Build history of the part. All positions in model axes, mm. Face numbers are marked on the shaded views. Coordinates: 2 decimals unless noted, no trailing zeros. Return JSON: item names as keys, results as strings.
from build123d import *

# Parameters (mm, degrees)
F0_R     = 2
F1_DEPTH = 15
F2_R     = 2
F3_SIZE2 = 0.334
F3_SIZE  = 0.167
F4_R     = 0.5
F5_SIZE  = 0.334


with BuildPart() as f1:
    # F0 (on Top) → F1 (new body)
    with BuildSketch(Plane.XY):
        with BuildLine():
            ThreePointArc((0, 7.5), (6.509248113, 3.7255454638), (6.4667999415, -3.7987495992))
            Line((6.4667999415, -3.7987495992), (7.3290399337, -4.3052495457))
            ThreePointArc((7.3290399337, -4.3052495457), (8.4999852198, -0.0158512782), (7.3450462726, 4.2778844366))
            ThreePointArc((7.3450462726, 4.2778844366), (10.1862523655, 11.2386714824), (3.53743112, 7.7289443698))
            ThreePointArc((3.53743112, 7.7289443698), (1.8102448532, 8.304999312), (0, 8.5))
            Line((0, 8.5), (0, 7.5))
        make_face()
        with Locations((7.5, 8.2748819776)):
            Circle(F0_R, mode=Mode.SUBTRACT)
        with BuildLine():
            ThreePointArc((-6.4667999415, -3.7987495992), (-6.509248113, 3.7255454638), (0, 7.5))
            Line((0, 7.5), (0, 8.5))
            ThreePointArc((0, 8.5), (-1.8102448532, 8.304999312), (-3.53743112, 7.7289443698))
            ThreePointArc((-3.53743112, 7.7289443698), (-10.1862523655, 11.2386714824), (-7.3450462726, 4.2778844366))
            ThreePointArc((-7.3450462726, 4.2778844366), (-8.4999852198, -0.0158512782), (-7.3290399337, -4.3052495457))
            Line((-7.3290399337, -4.3052495457), (-6.4667999415, -3.7987495992))
        make_face()
        with Locations((-7.5, 8.2748819776)):
            Circle(F0_R, mode=Mode.SUBTRACT)
    extrude(amount=F1_DEPTH)

    # F2
    f2_edges = [f1.edges().sort_by_distance(p)[0] for p in [
        (7.345046, 4.277884, 7.5),
        (3.537431, 7.728944, 7.5),
        (-3.537431, 7.728944, 7.5),
        (-7.345046, 4.277884, 7.5),
    ]]
    fillet(f2_edges, radius=F2_R)

    # F3
    f3_edges = [f1.edges().sort_by_distance(p)[0] for p in [
        (8.431287, -1.078612, 0),
        (8.276969, 3.688682, 0),
        (6.89792, -4.052, 0),
        (10.186252, 11.238671, 0),
        (0, 7.5, 0),
        (2.859731, 8.598635, 0),
        (-6.89792, -4.052, 0),
        (0, 8.5, 0),
        (-8.431287, -1.078612, 0),
        (-2.859731, 8.598635, 0),
        (-8.276969, 3.688682, 0),
        (-10.186252, 11.238671, 0),
        (5.5, 8.274882, 0),
        (-9.5, 8.274882, 0),
    ]]
    f3_side = f1.faces().sort_by_distance((8.150047, -1.042633, 0))[0]
    chamfer(f3_edges, length=F3_SIZE, length2=F3_SIZE2, reference=f3_side)

    # F4
    f4_edges = [f1.edges().sort_by_distance(p)[0] for p in [
        (-7.32904, -4.30525, 7.667),
        (7.32904, -4.30525, 7.667),
    ]]
    fillet(f4_edges, radius=F4_R)

    # F5
    f5_edges = [f1.edges().sort_by_distance(p)[0] for p in [
        (8.460888, -0.814478, 15),
        (7.278526, -4.092712, 15),
        (8.276969, 3.688682, 15),
        (6.675617, -3.921414, 15),
        (10.186252, 11.238671, 15),
        (0, 7.5, 15),
        (2.859731, 8.598635, 15),
        (-6.675617, -3.921414, 15),
        (0, 8.5, 15),
        (-7.278526, -4.092712, 15),
        (-2.859731, 8.598635, 15),
        (-8.460888, -0.814478, 15),
        (-10.186252, 11.238671, 15),
        (-8.276969, 3.688682, 15),
        (5.5, 8.274882, 15),
        (-9.5, 8.274882, 15),
    ]]
    chamfer(f5_edges, length=F5_SIZE)


solid = f1.part
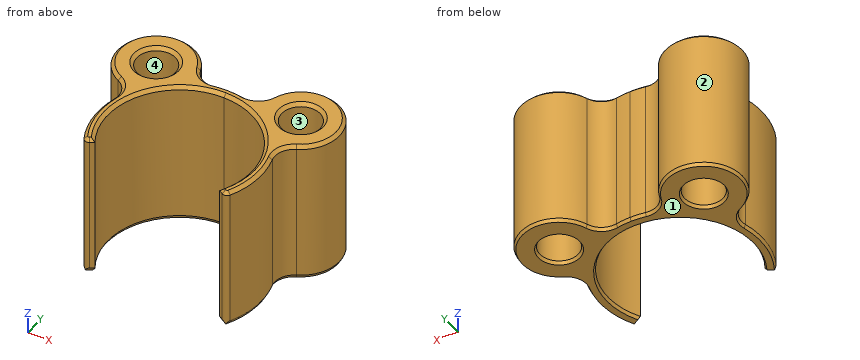
1. Probe L1, parallel to X at y = 11.75, z = 13.5; L2, parallel to X at y = 11.5, z = 7.5; L3, parallel to Y at x = 2.5, z = 12. List the from-to ranges inside material, lowest first.
Check values:
{"L1": "-9.48 to -5.52, 5.52 to 9.48", "L2": "-9.87 to -5.13, 5.13 to 9.87", "L3": "7.07 to 8.44"}
2. Drop flat-ended pins along their axis: pin 1 (1 mm diameter, centred on x = 1, z = 7, fed in from +Y); pin 2 (6 mm diameter, centred on x = -5.5, y = 9, fed in from +Z); pin 3 (3.5 mm diameter, centred on x = -7.5, y = 8.27, fed in from +Z). Give the stop position or say it passes through.
Check values:
{"pin 1": "y = 8.49", "pin 2": "z = 15", "pin 3": "through"}
3. Mould opens along Y. For the marked faces 1, 2, 3 and 4 say: pulls with the +Y half, pulls with the -Y half, needs draft (parallel to the pull), parting line crosses it, or undercut.
Check values:
{"face 1": "needs draft", "face 2": "parting line crosses it", "face 3": "undercut", "face 4": "undercut"}
4. Cut at A-A on z = 3.5. State how many separate pieces and enclosed holes the cut face has, plus the area to 3 significant figures.
Check values:
{"separate pieces": "1", "enclosed holes": "2", "area": "103 mm²"}
